Autodesk Inventor part; units mm, degrees
ref_plane "YZ Plane" through (0, 0, 0) normal (1, 0, 0) x (0, 1, 0)
ref_plane "XZ Plane" through (0, 0, 0) normal (0, 1, 0) x (-1, 0, 0)
ref_plane "XY Plane" through (0, 0, 0) normal (0, 0, 1) x (1, 0, 0)
sketch "Szkic1" plane through (0, 0, 0) normal (0, 1, 0) x (-1, 0, 0)
  line L0 (3, 18.5) -> (-6.25, 18.5)
  line L1 (-6.25, 18.5) -> (-6.25, 15.5)
  line L2 (-6.25, 15.5) -> (0, 15.5)
  line L3 (0, 15.5) -> (0, -15.5)
  line L4 (0, -15.5) -> (-6.25, -15.5)
  line L5 (-6.25, -15.5) -> (-6.25, -18.5)
  line L6 (-6.25, -18.5) -> (3, -18.5)
  line L7 (3, -18.5) -> (3, 18.5)
  line L8 (3, 0) -> (0, 0) construction
  line L9 (0, 3.9) -> (-2.5, 3.9)
  line L10 (-2.5, 3.9) -> (-2.5, 8)
  line L11 (-2.5, 8) -> (-2.5, 8)
  line L12 (-2.5, 8) -> (-6.25, 4.25)
  line L13 (-6.25, 4.25) -> (-6.25, -4.25)
  line L14 (-6.25, -4.25) -> (-2.5, -8)
  line L15 (-2.5, -8) -> (-2.5, -8)
  line L16 (-2.5, -8) -> (-2.5, -3.9)
  line L17 (-2.5, -3.9) -> (0, -3.9)
  line L18 (-2.5, 3.9) -> (-2.5, -3.9) construction
  line L19 (-2.5, 0) -> (-6.25, 0) construction
  line L20 (3, 18.5) -> (3, 15.5)
  line L21 (3, -15.5) -> (3, -18.5)
  line L22 (3, -18.5) -> (3, 18.5)
  circle A0 centre (30, 0) radius 7.75
  circle A1 centre (30, 0) radius 6.75
  line L23 (3, 18.5) -> (23.8501, 4.7161)
  line L24 (22.6643, 2.5) -> (3, 15.5)
  line L25 (3, -15.5) -> (22.6643, -2.5)
  line L26 (3, -18.5) -> (23.8501, -4.7161)
  line L27 (22.6643, 2.5) -> (3, 2.5)
  line L28 (22.6643, -2.5) -> (3, -2.5)
  point P0 (0, 0)
  point P1 (1.5, -15)
  point P2 (1.5, 18)
  point P3 (1.5, 0)
  point P4 (3, 2.5)
  dimension "d1" = 7.8
  dimension "d3" = 16
  dimension "d4" = 2.5
  dimension "d6" = 3
  dimension "d7" = 3
  dimension "d11" = 8.5
  dimension "d12" = 6.25
  dimension "d26" = 31
  dimension "d42" = 13.5
  dimension "d43" = 15.5
  dimension "d44" = 30
  dimension "d45" = 5
extrude "Wyciągnięcie proste2" add sketch "Szkic1" along normal blind 40 contours L7 L6 L5 L4 L3 L2 L1 L0 | L23 A0 L24 L7 | A0 | L27 A0 L28 L7 | A0 L26 L7 L25 | L3 L17 L16 L14 L13 L12 L10 L9
extrude "Wyciągnięcie proste7" cut sketch "Szkic1" along normal blind 38 contours L23 A0 L24 L7 | L27 A0 L28 L7 | A0 L26 L7 L25
extrude "Wyciągnięcie proste8" add sketch "Szkic1" along normal blind 2 contours L23 A0 L24 L7 | L27 A0 L28 L7 | A0 L26 L7 L25
properties part number "laser-solo"
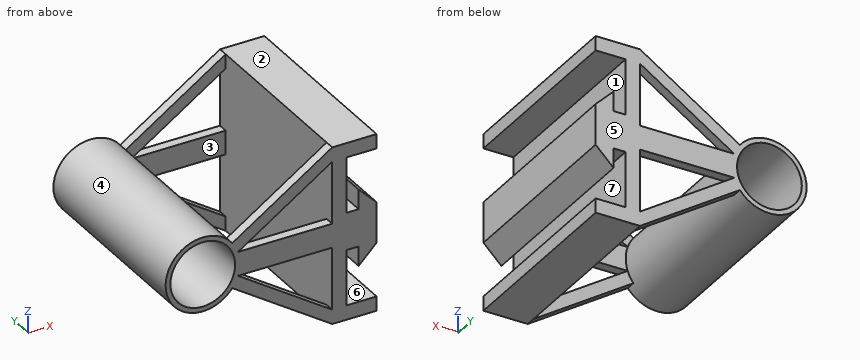
Could you check a few things on this model? Use its own coordinates, in mm. Face numbers are marked on the shaded views. A direction names the side the tool comes from. Give positions to 0.01 mm unless a question says otherwise; leave off trailing zeros. Order: outer loops, then holes, each group sorted by start corner. A loop starts at its lowest first (then second) coordinate and runs counter-clockwise, first axis right, second up.
Q1. I'm going to push flat-ended pins straight in: P1, Ø1.2, axis at y = 18.5, z = 5.5, coming from the -X side; P2, Ø1, axis at x = -13, y = 39, coming from the -Z side; P3, Ø6, axis at y = 20, z = -5, coming from the -X side. Where does each tip first touch, or does it pass through?
Q2. For the marked faces 5, 6 and 7, which set-ups out of +Z, -Z, +X, -X, +Y, -Y let a thin tool reach every point of the face, with its end or its side?
Q3. We'd pull the mould along Z, two halves only. Please class the marked faces 1, 2, 3 and 4: +Z half, -Z half, draft (parallel to the pull), parting line (faces both ways), or undercut.
Q4. Suppose I cut it at B-B, the plane x = -30. Write out the boundary of the cut face in (y, z).
Q5. Suppose I cut it at D-D, the plane z = -13.5. Write out the boundary of the cut face in (x, y).
Q6. If I drill on line 1 along Z through (x, y) = (-30, 26); line 2 along X through (y, z) = (38.5, 6); line 3 along Z through (x, y) = (4, 27), over which ranges is the centre line in solid material (lowest first)?
Q7. Suppose I cut it at A-A, the plane z = 0. Write out the boundary of the cut face in (x, y), and give its area (3 significant figures).
Q8. Suppose I cut it at C-C, the plane y = 8. Write out the boundary of the cut face in (x, z), and give its area (3 significant figures).
Solution:
1. P1: stops at x = -36
1. P2: stops at z = -12.22
1. P3: stops at x = -37.49
2. face 5: +Z, -Z, +X, -X, +Y
2. face 6: +X, +Y, -Y
2. face 7: +Y, -Y
3. face 1: undercut
3. face 2: +Z half
3. face 3: draft
3. face 4: parting line
4. outline: (0, -7.75) - (40, -7.75) - (40, -6.75) - (0, -6.75) - close; (0, 6.75) - (40, 6.75) - (40, 7.75) - (0, 7.75) - close
5. outline: (-10.56, 0) - (-6.03, 0) - (-6.03, 2) - (-10.56, 2) - close; (-10.56, 38) - (-6.03, 38) - (-6.03, 40) - (-10.56, 40) - close; (-3, 0) - (0, 0) - (0, 40) - (-3, 40) - close
6. line 1: z = -7.75 to -6.75, 6.75 to 7.75
6. line 2: x = -34.91 to -33.09, -26.91 to -25.09, -21.91 to -17.37, -3 to 0, 2.5 to 4.5
6. line 3: z = -18.5 to -15.5, -6.5 to 6.5, 15.5 to 18.5
7. outline: (-37.75, 0) - (-36.75, 0) - (-36.75, 40) - (-37.75, 40) - close; (-23.25, 0) - (6.25, 0) - (6.25, 40) - (-23.25, 40) - close; hole (-22.25, 2) - (-3, 2) - (-3, 38) - (-22.25, 38) - close
7. area: 527 mm2
8. outline: circle Ø15.5 at (-30, 0); (-3, -18.5) - (6.25, -18.5) - (6.25, -15.5) - (0, -15.5) - (0, -3.9) - (2.5, -3.9) - (2.5, -8) - (6.25, -4.25) - (6.25, 4.25) - (2.5, 8) - (2.5, 3.9) - (0, 3.9) - (0, 15.5) - (6.25, 15.5) - (6.25, 18.5) - (-3, 18.5) - close; hole circle Ø13.5 at (-30, 0)
8. area: 259 mm2
